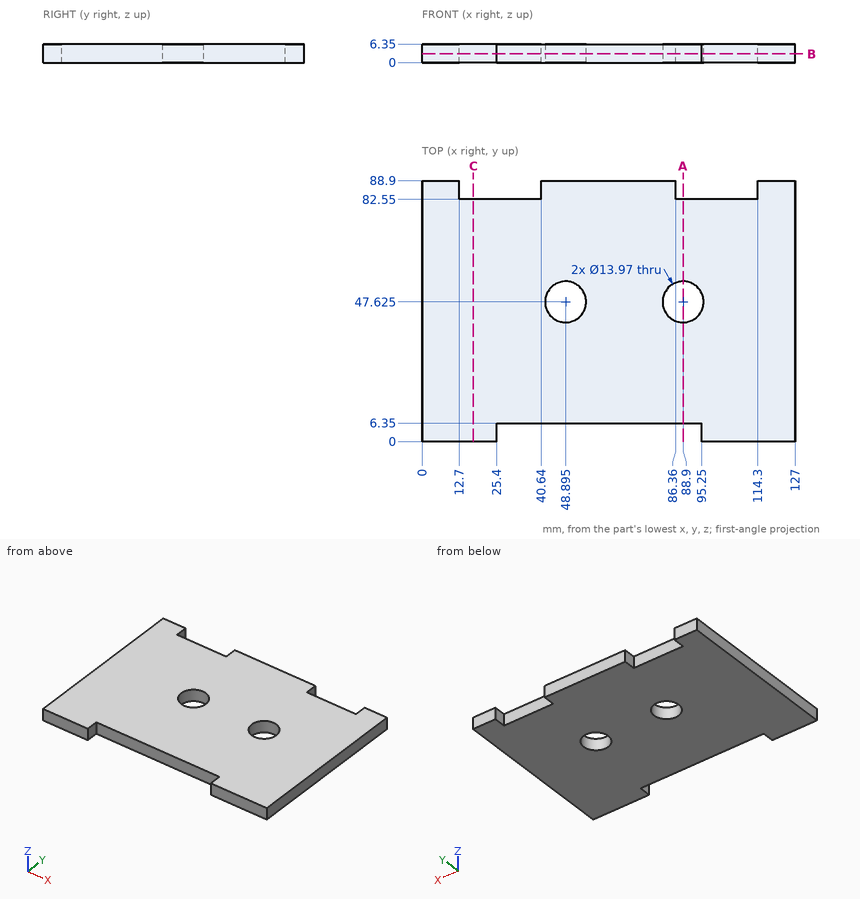
Part print with two shaded views. Sizes in mm from the minimum x, y, z corner. Round coordinates to 2 decimals unless told otherwise and drop trailing zeros. Loops run counter-clockwise (first coordinate to the right, second up) from the corner with the lowest first, then second, coordinate; pieces in that order, holes last. Notation, with made-up numbers: M -9.5,29 L 11.5,29 A28 cw 11.5,52 Z; hole C -2.75,62 d6. An arc over 180 degrees is marked long. Return JSON: item names as keys, results as strings. Group by question number.
(1) Saw through at C-C, the plane x = 17.5. List the corners of the cut face in (y, z).
(2) Saw through at A-A, the plane x = 88.9. List the corners of the cut face in (y, z).
(3) Saw through at B-B, the plane z = 3. List the corners of the cut face in (x, y) (3 decimals), and give its area (3 significant figures).
(4) Wall check: probe 1 along Y at (x, z) = (88.5, 4.25); probe 2 along Y at (x, z) = (88.9, 2.5); probe 3 along Y at (x, z) = (38, 1.5). Give the ranges that are in metal, low to high. Write a range as [from, to].
(5) Drop flat-ended pins along their axis: P1, Ø3, axis at x = 71, z = 4.5, coming from the -Y side; P2, Ø3, axis at x = 25.5, z = 3.5, coming from the +Y side. Give the stop position or say it passes through.
Answer list:
{
 "1": {"outline": "M 0,0 L 82.55,0 L 82.55,6.35 L 0,6.35 Z"},
 "2": {"outline": "M 6.35,0 L 40.64,0 L 40.64,6.35 L 6.35,6.35 Z; M 54.61,0 L 82.55,0 L 82.55,6.35 L 54.61,6.35 Z"},
 "3": {"outline": "M 0,0 L 25.4,0 L 25.4,6.35 L 95.25,6.35 L 95.25,0 L 127,0 L 127,88.9 L 114.3,88.9 L 114.3,82.55 L 86.36,82.55 L 86.36,88.9 L 40.64,88.9 L 40.64,82.55 L 12.7,82.55 L 12.7,88.9 L 0,88.9 Z; hole C 48.895,47.625 d13.97; hole C 88.9,47.625 d13.97", "area": "10,200 mm2"},
 "4": {"probe 1": "[6.35, 40.65], [54.6, 82.55]", "probe 2": "[6.35, 40.64], [54.61, 82.55]", "probe 3": "[6.35, 82.55]"},
 "5": {"P1": "y = 6.35", "P2": "y = 82.55"}
}
